```python
from build123d import *

# Parameters (mm, degrees)
SKETCH1_R           = 22.5
BOSS_EXTRUDE1_DEPTH = 100
SKETCH2_W           = 14
SKETCH2_H           = 8.804237579
CUT_EXTRUDE1_DEPTH  = 105.940459309
CHAMFER1_SIZE       = 2


with BuildPart() as part:
    # Sketch1 → Boss-Extrude1 (new body)
    with BuildSketch(Plane.XY):
        Circle(SKETCH1_R)
    extrude(amount=BOSS_EXTRUDE1_DEPTH)

    # Sketch2 → Cut-Extrude1 (cut, through all)
    with BuildSketch(Plane.XY.offset(100)):
        with Locations((0, 21.90211879)):
            Rectangle(SKETCH2_W, SKETCH2_H)
    extrude(amount=-CUT_EXTRUDE1_DEPTH, mode=Mode.SUBTRACT)

    # Chamfer1
    chamfer1_edges = [part.edges().sort_by_distance(p)[0] for p in [
        (7, 19.44170239, 100),
        (-7, 19.44170239, 100),
        (0, 17.5, 100),
        (0, -22.5, 100),
    ]]
    chamfer(chamfer1_edges, length=CHAMFER1_SIZE)


solid = part.part
```
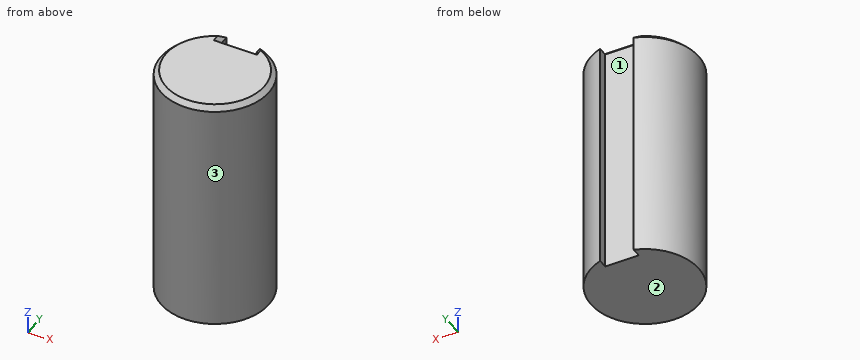
Part model, mm, in its own coordinate system. Face numbers are marked on the shaded views. Round coordinates to 2 decimals unless told otherwise and drop trailing zeros. Write each loop counter-clockwise with the first axis right and the second up, starting at its lowest first coordinate (ties: lowest second). Pieces come first, ordered by that corner, then holes.
Item 1: Cut at A-A, the plane x = 0. Give the cut face in (y, z).
Results:
outline: (-22.5, 0) - (17.5, 0) - (17.5, 98) - (15.5, 100) - (-20.5, 100) - (-22.5, 98) - close
Item 2: Drop flat-ended pins along their axis: pin 1 Ø2 at (y, z) = (-11.5, 83.5) entering from -X; pin 2 Ø4 at (y, z) = (9, 60.5) entering from +X; pin 3 Ø1 at (x, z) = (-14.5, 47) entering from +Y; pin 4 Ø10 at (y, z) = (-1.5, 63.5) entering from -X. Give the stop position or say it passes through.
Results:
pin 1: stops at x = -19.9
pin 2: stops at x = 21.38
pin 3: stops at y = 17.61
pin 4: stops at x = -22.5
Item 3: Probe L1, parallel to X at y = 19, z = 89; L2, parallel to X at y = 19.5, z = 79.5; L3, parallel to X at y = -19.5, z = 93. List the from-to ranges inside material, lowest first.
Results:
L1: x = -12.05 to -7, 7 to 12.05
L2: x = -11.22 to -7, 7 to 11.22
L3: x = -11.22 to 11.22
Item 4: Cut at B-B, the plane z = 93. Give the cut face in (x, y).
Results:
outline: (-7, 17.5) - (-7, 21.38) arc R22.5 ccw (long way) to (7, 21.38) - (7, 17.5) - close
Item 5: Two-plate mould, pull along X, no slides. Class the marked faces 1, 2 and 3: +X half, -X half, draft (parallel to the pull), parting line (faces both ways), or undercut.
Results:
face 1: undercut
face 2: draft
face 3: parting line
